Geometry: see drawing. Coordinates: mm, zero at the bounding-box minimum. A direction names the side the tool comes from. Coordinates: 2 decimals unless noted, no trailing zeros. Write each loop counter-clockwise with the first axis right and the second up, starting at its lowest first coordinate (ties: lowest second). Pieces come first, ordered by that corner, then holes.
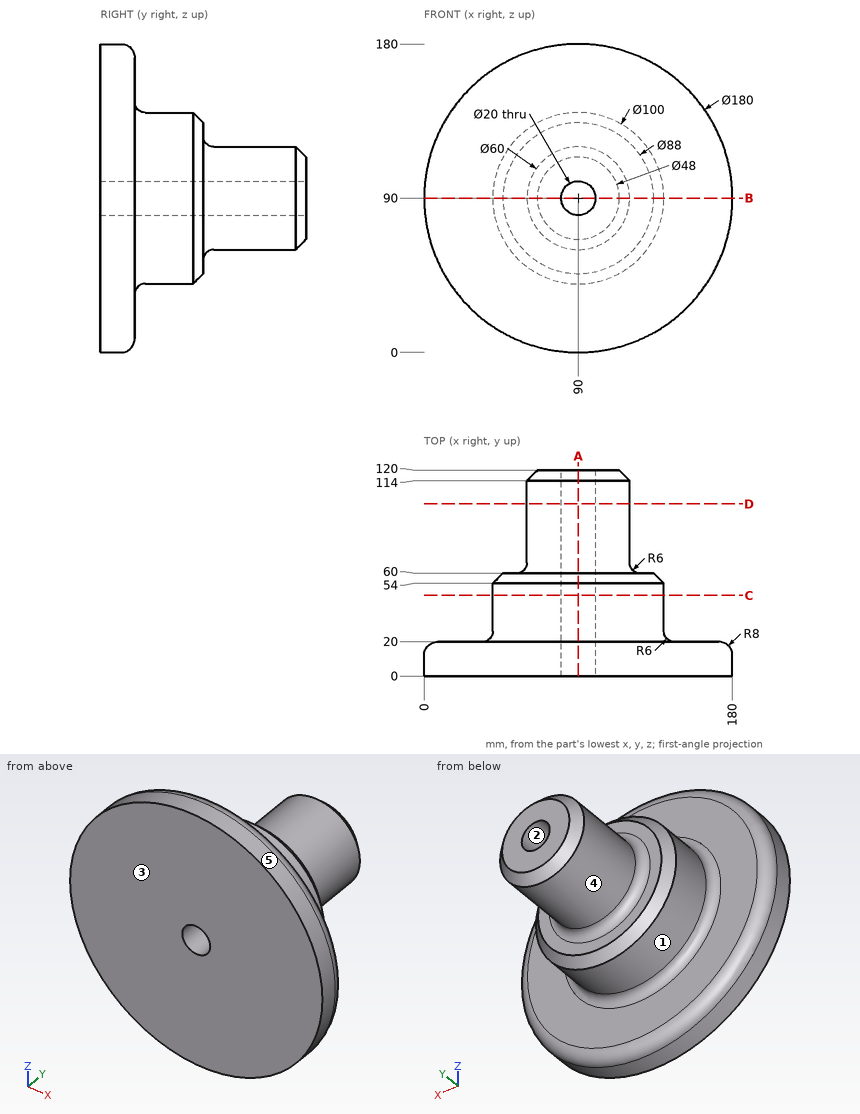
Item 1: Material intervals for probe 1 along Z at (x, y) = (90, 71.5); probe 2 along Z at (x, y) = (90, 31); probe 3 along Y at (x, z) = (35, 72), sorted ascending.
Derived:
probe 1: z = 60 to 80, 100 to 120
probe 2: z = 40 to 80, 100 to 140
probe 3: y = 0 to 20
Item 2: Section D-D, the plane y = 100.5. Output: boundary loops of the cut face in (x, z).
Derived:
outline: circle Ø60 at (90, 90); hole circle Ø20 at (90, 90)
Item 3: Pull-direction query (X, two-part tool) for the marked faces 1, 2 and 3; classes: released by +X, released by -X, zero draft, split by the parting line, or undercut.
Derived:
face 1: split by the parting line
face 2: undercut
face 3: zero draft
Item 4: Section A-A, the plane x = 90. Output: boundary loops of the cut face in (y, z).
Derived:
outline: (0, 0) - (12, 0) arc R8 ccw to (20, 8) - (20, 34) arc R6 cw to (26, 40) - (54, 40) - (60, 46) - (60, 54) arc R6 cw to (66, 60) - (114, 60) - (120, 66) - (120, 80) - (0, 80) - close; (0, 100) - (120, 100) - (120, 114) - (114, 120) - (66, 120) arc R6 cw to (60, 126) - (60, 134) - (54, 140) - (26, 140) arc R6 cw to (20, 146) - (20, 172) arc R8 ccw to (12, 180) - (0, 180) - close
Item 5: Section C-C, the plane y = 47. Output: boundary loops of the cut face in (x, z), plus the area to 3 significant figures.
Derived:
outline: circle Ø100 at (90, 90); hole circle Ø20 at (90, 90)
area: 7,540 mm2
Item 6: Section B-B, the plane z = 90. Output: boundary loops of the cut face in (x, y).
Derived:
outline: (0, 0) - (80, 0) - (80, 120) - (66, 120) - (60, 114) - (60, 66) arc R6 cw to (54, 60) - (46, 60) - (40, 54) - (40, 26) arc R6 cw to (34, 20) - (8, 20) arc R8 ccw to (0, 12) - close; (100, 0) - (180, 0) - (180, 12) arc R8 ccw to (172, 20) - (146, 20) arc R6 cw to (140, 26) - (140, 54) - (134, 60) - (126, 60) arc R6 cw to (120, 66) - (120, 114) - (114, 120) - (100, 120) - close
Item 7: Set-up query: the marked faces 4 and 5. Return all of +Z, -Z, +X, -X, +Y, -Y with unobstructed straight access to the full face (end or side cutting, diameter ignored); none if empty.
Derived:
face 4: +Y
face 5: +Y, -Y
Item 8: Pin query (flat end, axial travel): pin 1 (4 mm diameter, centred on x = 95.5, z = 62.5, fed in from +Y); pin 2 (1.5 mm diameter, centred on x = 101, y = 27.5, fed in from -Z); pin 3 (12 mm diameter, centred on x = 120, y = 51.5, fed in from -Z). Return the tip coordinate at first contact, or that it passes through.
Derived:
pin 1: stops at y = 117.96
pin 2: stops at z = 41.06
pin 3: stops at z = 46.14
